Study the drawing (mm; zero at the part's minimum x, y, z) and answer. Give positions to 0.01 mm unless a question says otherwise; leave off trailing zeros. Loops run counter-clockwise (first coordinate to the right, second up) from the corner with the lowest first, then second, coordinate; pieces in that order, holes last. Notation, with made-up numbers: M 59,85 L 87,85 A17 ccw 87,106 Z; hole C -7,66 d10. An arc over 180 degrees is marked long. Use one line per item in the form item = value. Start each with the question number.
1. The part is cut by section B-B (z = 5). Write down the section's boundary in (x, y).
2. This flat-tipped pin is pushed along its axis until it touches: pin 1 Ø1.5 at (y, z) = (2, 25) entering from -X. Where does it stop, or does it pass through?
3. The part is cut by section C-C (y = 5.25). Write down the section's boundary in (x, z), and give its area (3 significant figures).
4. Straight lines are drawn through the part: line 1 (X direction, y = 7.25, z = 15); line 2 (Z direction, x = 15, y = 3); line 3 (Z direction, x = 4, y = 7.75). For each, find the intervals that lie inside material, in ascending order. Write a range as from..to.
5. The part is cut by section A-A (x = 15). Write down the section's boundary in (y, z), and give its area (3 significant figures).
6. The part is cut by section D-D (x = 5.75). Write down the section's boundary in (y, z).
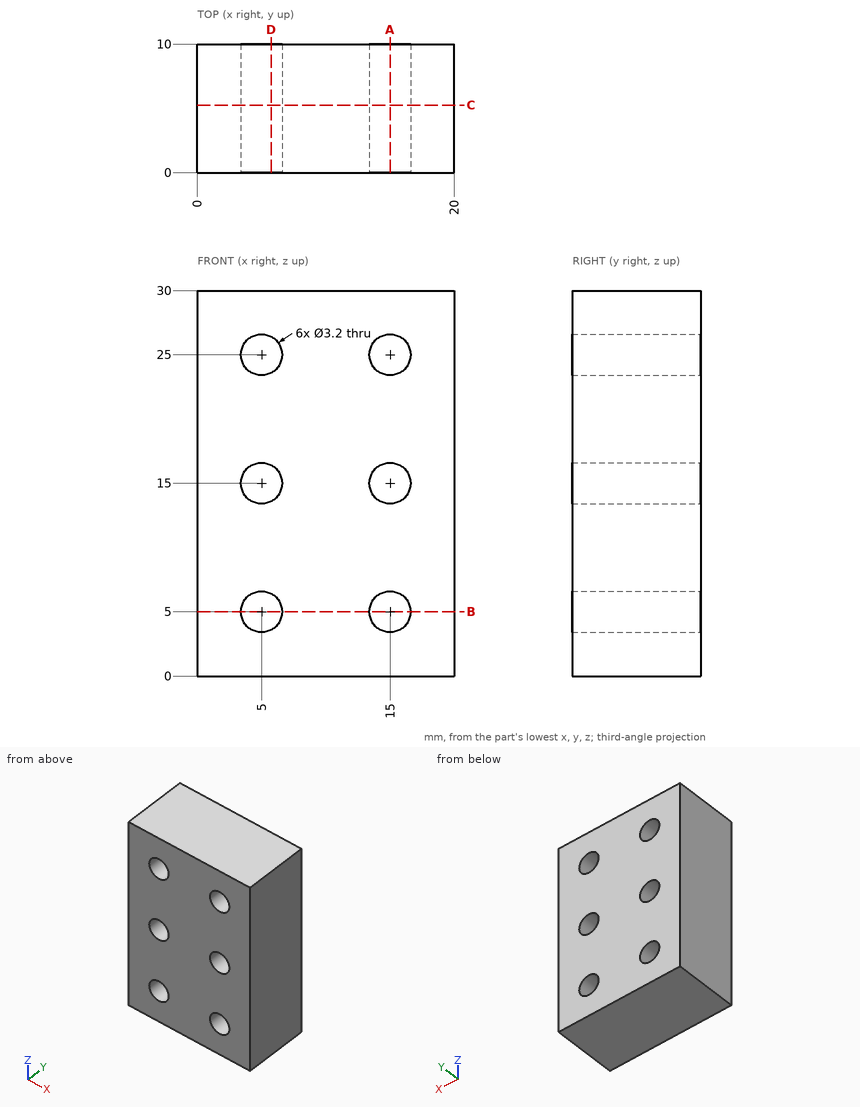
Derived:
q1.outline = M 0,0 L 3.4,0 L 3.4,10 L 0,10 Z; M 6.6,0 L 13.4,0 L 13.4,10 L 6.6,10 Z; M 16.6,0 L 20,0 L 20,10 L 16.6,10 Z
q2.pin_1 = 0
q3.outline = M 0,0 L 20,0 L 20,30 L 0,30 Z; hole C 5,5 d3.2; hole C 5,15 d3.2; hole C 5,25 d3.2; hole C 15,5 d3.2; hole C 15,15 d3.2; hole C 15,25 d3.2
q3.area = 552 mm2
q4.line_1 = 0..3.4, 6.6..13.4, 16.6..20
q4.line_2 = 0..3.4, 6.6..13.4, 16.6..23.4, 26.6..30
q4.line_3 = 0..3.75, 6.25..13.75, 16.25..23.75, 26.25..30
q5.outline = M 0,0 L 10,0 L 10,3.4 L 0,3.4 Z; M 0,6.6 L 10,6.6 L 10,13.4 L 0,13.4 Z; M 0,16.6 L 10,16.6 L 10,23.4 L 0,23.4 Z; M 0,26.6 L 10,26.6 L 10,30 L 0,30 Z
q5.area = 204 mm2
q6.outline = M 0,0 L 10,0 L 10,3.59 L 0,3.59 Z; M 0,6.41 L 10,6.41 L 10,13.59 L 0,13.59 Z; M 0,16.41 L 10,16.41 L 10,23.59 L 0,23.59 Z; M 0,26.41 L 10,26.41 L 10,30 L 0,30 Z
